```python
from build123d import *

# Parameters (mm, degrees)
SKETCH2_R           = 3.175
BOSS_EXTRUDE1_DEPTH = 2.38125
SKETCH3_R           = 3.57124
BOSS_EXTRUDE2_DEPTH = 9.525
SKETCH5_R           = 3.175
BOSS_EXTRUDE3_DEPTH = 4.7625


with BuildPart() as part:
    # Sketch2 → Boss-Extrude1 (new, symmetric)
    with BuildSketch(Plane(origin=(0, 0, 0), x_dir=(0, 0, -1), z_dir=(1, 0, 0))):
        with Locations(Location((0, 0, 0), (0, 0, 180))):
            Circle(SKETCH2_R)
    extrude(amount=BOSS_EXTRUDE1_DEPTH, both=True)

    # Sketch3 → Boss-Extrude2 (add)
    with BuildSketch(Plane.ZY.offset(2.38125)):
        with Locations(Location((0, 0, 0), (0, 0, 180))):
            Circle(SKETCH3_R)
    extrude(amount=BOSS_EXTRUDE2_DEPTH)

    # Sketch5 → Boss-Extrude3 (add)
    with BuildSketch(Plane.ZY.offset(11.90625)):
        Circle(SKETCH5_R)
    extrude(amount=BOSS_EXTRUDE3_DEPTH)


solid = part.part
```
Check sheet for the modelled part. Datum: model origin and axes. Units: mm. A direction names the side the tool comes from. Give positions to 0.01 mm unless a question says otherwise; leave off trailing zeros. Order: outer loops, then holes, each group sorted by start corner. A loop starts at its lowest first (then second) coordinate and runs counter-clockwise, first axis right, second up. Notation, with made-up numbers: M 53.5,3.5 L 95.5,3.5 A18 ccw 95.5,16.5 Z; hole C 33.25,43 d9. An arc over 180 degrees is marked long. Answer in a Markdown table with one row per item. Add a question column.
Q1. Sectioned sample at C-C, the plane x = -13.75. Record the boundary of the cut face in (y, z) (3 decimals).
Q2. Sectioned sample at A-A, the plane y = 0. Record the boundary of the cut face in (x, z) (3 decimals), and give its area (3 significant figures).
Q3. Access from +Z, -Z, +X, -X, +Y, -Y to the whole of each face (thin tool, end or side, straight path). Record for faces 1 (the cylindrical face through (-14.25, -3.1, -0.69)), 2 (the flat face through (2.381, 0, 0)), 3 (the cylindrical face through (0, 2.8, 1.5)).
Q4. Gauge pin test, flat end, axial feed: pin 1 Ø1.5 at (y, z) = (-2, -2.5) entering from +X. Record the tip position at first contact, or that the pin passes through.
Q5. Thickness scan on L1, parallel to X at y = -1, z = 3.25; L2, parallel to Z at x = 1.75, y = 1.5; L3, parallel to Y at x = -0.25, z = 0 (3 decimals). Record the ranges inside material, lowest first.
Q6. Sectioned sample at D-D, the plane x = -10.75. Record the boundary of the cut face in (y, z), and give its area (3 significant figures).
Verdict:
| question | item | result |
|---|---|---|
| 1 | outline | C 0,0 d6.35 |
| 2 | outline | M -16.669,-3.175 L -11.906,-3.175 L -11.906,-3.571 L -2.381,-3.571 L -2.381,-3.175 L 2.381,-3.175 L 2.381,3.175 L -2.381,3.175 L -2.381,3.571 L -11.906,3.571 L -11.906,3.175 L -16.669,3.175 Z |
| 2 | area | 129 mm² |
| 3 | face 1 | -X |
| 3 | face 2 | +Z, -Z, +X, +Y, -Y |
| 3 | face 3 | +X |
| 4 | pin 1 | x = 2.38 |
| 5 | L1 | -11.91 to -2.38 |
| 5 | L2 | -2.8 to 2.8 |
| 5 | L3 | -3.175 to 3.175 |
| 6 | outline | C 0,0 d7.14 |
| 6 | area | 40.1 mm² |
